from build123d import *

# Parameters (mm, degrees)
F0_W     = 44
F0_H     = 25.4
F1_DEPTH = 77.5
F3_W     = 63
F3_H     = 50.5
F3_R     = 2.5
F2_W     = 44
F2_H     = 77.5
F4_DEPTH = 10


with BuildPart() as f1:
    # F0 (on Front) → F1 (new body)
    with BuildSketch(Plane.XZ):
        Rectangle(F0_W, F0_H)
    extrude(amount=-F1_DEPTH)

    # F3 (on face) + F2 (on face) → F4 (join)
    with BuildSketch(Plane.XY.offset(12.7)):
        with Locations((0, 38.75)):
            Rectangle(F3_W, F3_H)
        with Locations((-26.5, 18.75)):
            Circle(F3_R, mode=Mode.SUBTRACT)
        with Locations((26.5, 18.75)):
            Circle(F3_R, mode=Mode.SUBTRACT)
        with Locations((-26.5, 58.75)):
            Circle(F3_R, mode=Mode.SUBTRACT)
        with Locations((26.5, 58.75)):
            Circle(F3_R, mode=Mode.SUBTRACT)
    with BuildSketch(Plane.XY.offset(12.7)):
        with Locations((0, 38.75)):
            Rectangle(F2_W, F2_H)
    extrude(amount=-F4_DEPTH)


solid = f1.part
The model under review builds one solid part; all positions refer to its coordinate system, in mm. A direction names the side the tool comes from. Round coordinates to 2 decimals unless told otherwise and drop trailing zeros. Loops run counter-clockwise (first coordinate to the right, second up) from the corner with the lowest first, then second, coordinate; pieces in that order, holes last. Notation, with made-up numbers: (84.5, 9) - (103.5, 9) arc R24 cw to (103.5, 43) - close; hole circle Ø9 at (7, 70). An arc over 180 degrees is marked (long way). Use CSV: the item, a comma, the result in double quotes.
(1) For line 1 (Y direction, x = 26.5, z = 8.75); line 2 (X direction, y = 35, z = -2.5); line 3 (Z direction, x = 22.5, y = 32), list the stretches that pass through material, from the lowest coordinate up.
Working result:
line 1,"y = 13.5 to 16.25, 21.25 to 56.25, 61.25 to 64"
line 2,"x = -22 to 22"
line 3,"z = 2.7 to 12.7"
(2) Machinability: for faces 5 (the flat face through (-27, 13.5, 8)), 6 (the flat face through (-27, 64, 8)), 7 (the flat face through (27, 39, 2.7)), 8 (the flat face through (-27, 39, 2.7)), which of the approach directions +Z, -Z, +X, -X, +Y, -Y give a long, thin tool a straight path to every point of the face, cutting with its end or side? Answer none if there is none.
Working result:
face 5,"+Z, -Z, -X, -Y"
face 6,"+Z, -Z, -X, +Y"
face 7,"-Z, +X, +Y, -Y"
face 8,"-Z, -X, +Y, -Y"
(3) Take a section at C-C, the plane z = 7.25. Give the boundary of the cut face in (x, y), plus the area to 3 significant figures.
Working result:
outline,"(-31.5, 13.5) - (-22, 13.5) - (-22, 0) - (22, 0) - (22, 13.5) - (31.5, 13.5) - (31.5, 64) - (22, 64) - (22, 77.5) - (-22, 77.5) - (-22, 64) - (-31.5, 64) - close; hole circle Ø5 at (-26.5, 18.75); hole circle Ø5 at (-26.5, 58.75); hole circle Ø5 at (26.5, 18.75); hole circle Ø5 at (26.5, 58.75)"
area,"4,290 mm^2"
(4) The part is to be moulded in two halves that separate along Y. For faces 1 (the cylindrical face through (24.66, 60.44, 7.77)), 2 (the cylindrical face through (26.17, 21.23, 7.77)), 3 (the flat face through (27, 64, 8)), 4 (the flat face through (22, 38, -3)), say which applies: pulls with the +Y half, pulls with the -Y half, needs draft (parallel to the pull), parting line crosses it, or undercut.
Working result:
face 1,"undercut"
face 2,"undercut"
face 3,"pulls with the +Y half"
face 4,"needs draft"
(5) Take a section at D-D, the plane x = -25. Give the boundary of the cut face in (y, z).
Working result:
outline,"(13.5, 2.7) - (16.75, 2.7) - (16.75, 12.7) - (13.5, 12.7) - close; (20.75, 2.7) - (56.75, 2.7) - (56.75, 12.7) - (20.75, 12.7) - close; (60.75, 2.7) - (64, 2.7) - (64, 12.7) - (60.75, 12.7) - close"
(6) Clearance check with flat-ended pins moving along their axes: P1, Ø5, axis at x = 26, y = 35, coming from the -Z side; P2, Ø7.5, axis at x = 27.5, z = 6, coming from the -Y side; P3, Ø10.5, axis at x = -29, z = 5.5, coming from the +Y side. State where each tip first meets the part, or that it passes through.
Working result:
P1,"stops at z = 2.7"
P2,"stops at y = 13.5"
P3,"stops at y = 64"
(7) Take a section at A-A, the plane y = 58.75. Give the boundary of the cut face in (x, z), plus the area to 3 significant figures.
Working result:
outline,"(-31.5, 2.7) - (-29, 2.7) - (-29, 12.7) - (-31.5, 12.7) - close; (-24, 2.7) - (-22, 2.7) - (-22, -12.7) - (22, -12.7) - (22, 2.7) - (24, 2.7) - (24, 12.7) - (-24, 12.7) - close; (29, 2.7) - (31.5, 2.7) - (31.5, 12.7) - (29, 12.7) - close"
area,"1,210 mm^2"
(8) Take a section at B-B, the plane x = 26.5. Give the boundary of the cut face in (y, z).
Working result:
outline,"(13.5, 2.7) - (16.25, 2.7) - (16.25, 12.7) - (13.5, 12.7) - close; (21.25, 2.7) - (56.25, 2.7) - (56.25, 12.7) - (21.25, 12.7) - close; (61.25, 2.7) - (64, 2.7) - (64, 12.7) - (61.25, 12.7) - close"
